Work out the finished part from the listing and answer in its coordinate system (mm). Face numbers are marked on the shaded views. A direction names the side the tool comes from. Coordinates: 2 decimals unless noted, no trailing zeros. Order: outer loops, then holes, each group sorted by start corner. A loop starts at its lowest first (then second) coordinate and runs counter-clockwise, first axis right, second up.
Autodesk Inventor part; units mm, degrees
ref_plane "YZ Plane" through (0, 0, 0) normal (1, 0, 0) x (0, 1, 0)
ref_plane "XZ Plane" through (0, 0, 0) normal (0, 1, 0) x (-1, 0, 0)
ref_plane "XY Plane" through (0, 0, 0) normal (0, 0, 1) x (1, 0, 0)
sketch "Sketch1" plane through (0, 0, 0) normal (0, 1, 0) x (-1, 0, 0)
  line L0 (0, 0) -> (1000, 0)
  line L1 (1000, 0) -> (1000, 1000)
  line L2 (1000, 1000) -> (0, 1000)
  line L3 (0, 1000) -> (0, 0)
  line L4 (-100, 1100) -> (1100, 1100)
  line L5 (1100, 1100) -> (1100, -100)
  line L6 (1100, -100) -> (-100, -100)
  line L7 (-100, -100) -> (-100, 1100)
  dimension "d0" = 1000
  dimension "d1" = 1000
  dimension "d2" = 100
extrude "Extrusion1" add sketch "Sketch1" along normal blind 850 contours L3 L2 L1 L0
extrude "Extrusion2" add sketch "Sketch1" along normal blind 10
sketch "Sketch2" plane through (0, 10, 0) normal (0, 1, 0) x (1, 0, 0)
  line L0 (100, 100) -> (-1100, 100)
  line L1 (-1100, 100) -> (-1100, -1100)
  line L2 (-1100, -1100) -> (100, -1100)
  line L3 (100, -1100) -> (100, 100)
  line L4 (0, -1000) -> (0, 0)
  line L5 (-1000, -1000) -> (0, -1000)
  line L6 (-1000, 0) -> (-1000, -1000)
  line L7 (0, 0) -> (-1000, 0)
  line L8 (-1000, -1000) -> (-1050, -1000)
  line L9 (-1050, -1000) -> (-1050, -1050)
  line L10 (-1050, -1050) -> (50, -1050)
  line L11 (50, -1050) -> (50, 50)
  line L12 (50, 50) -> (-1050, 50)
  line L13 (-1050, 50) -> (-500, 50)
  line L14 (-500, 50) -> (-500, -1050)
  line L15 (50, 50) -> (50, -500)
  line L16 (50, -500) -> (-1000, -500)
  line L17 (-1000, -500) -> (-1050, -500)
  dimension "d7" = 50
  dimension "d8" = 50
  dimension "d9" = 1100
  dimension "d10" = 1100
  dimension "d11" = 550
hole "Hole1" at (-1050, 10, 1050) at (-500, 10, 1050) at (50, 10, 1050) at (50, 10, -50) at (-500, 10, -50) at (-1050, 10, -50) at (50, 10, 500) at (-1050, 10, 500) direction (0, -1, 0) diameter 25.4 end through all
sketch "Sketch3" plane through (0, 850, 1000) normal (1, 0, 0) x (0, 0, -1)
  line L0 (0, -59.4954) -> (1000, -59.4954) construction
  line L1 (1000, -59.4954) -> (1000, -749.3909) construction
  line L2 (1000, -749.3909) -> (0, -749.3909) construction
  line L3 (0, -749.3909) -> (0, -59.4954) construction
  point P0 (1000, -850)
decal "Decal1"
sketch "Sketch4" plane through (-1000, 850, 1000) normal (0, 0, 1) x (1, 0, 0)
  line L0 (0, -840) -> (0, 0)
  line L1 (0, -64.0631) -> (1000, -64.0631) construction
  line L2 (1000, -64.0631) -> (1000, -753.9585) construction
  line L3 (1000, -753.9585) -> (0, -753.9585) construction
  line L4 (0, -753.9585) -> (0, -64.0631) construction
  point P0 (1000, -850)
decal "Decal2"
sketch "Sketch5" plane through (-1000, 850, 0) normal (-1, 0, 0) x (0, 0, 1)
  line L0 (57.8435, -18.5187) -> (921.1484, -18.5187) construction
  line L1 (921.1484, -18.5187) -> (921.1484, -825.537) construction
  line L2 (921.1484, -825.537) -> (57.8435, -825.537) construction
  line L3 (57.8435, -825.537) -> (57.8435, -18.5187) construction
  point P0 (0, -850)
decal "Decal3"
sketch "Sketch6" plane through (0, 850, 0) normal (0, 0, -1) x (-1, 0, 0)
  line L0 (-2.3743, -103.2912) -> (997.1946, -103.2912) construction
  line L1 (997.1946, -103.2912) -> (997.1946, -725.2451) construction
  line L2 (997.1946, -725.2451) -> (-2.3743, -725.2451) construction
  line L3 (-2.3743, -725.2451) -> (-2.3743, -103.2912) construction
  point P0 (0, -850)
decal "Decal4"
sketch "Sketch7" plane through (0, 0, 0) normal (0, -1, 0) x (1, 0, 0)
  circle A0 centre (-1050, 500) radius 12.7
  circle A1 centre (-500, 500) radius 5
  point P0 (0, 0)
  dimension "d73" = 10
extrude "Extrusion3" cut sketch "Sketch7" against normal blind 1 contours A1
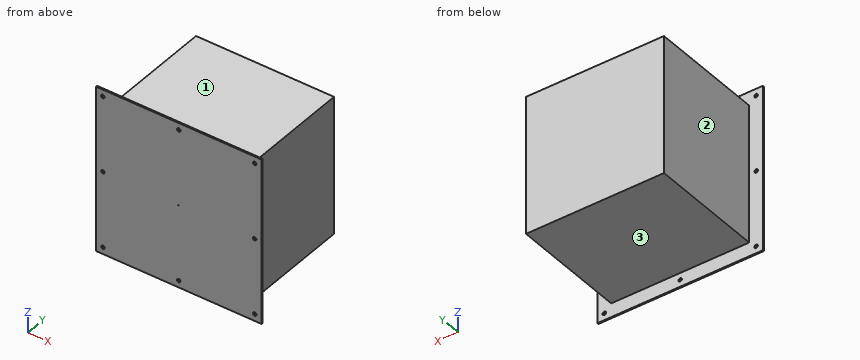
1. The part is cut by section B-B (x = -468.5). Determine the outline of the cut face in (y, z).
2. The part is cut by section A-A (z = 537). Determine the outline of the cut face in (x, y), plus the area to 3 significant figures.
3. The part is cut by section C-C (y = 680). Determine the outline of the cut face in (x, z).
4. Flat-ended cylindrical pins translate along their axes: pin 1 (5 mm diameter, centred on x = -500.5, z = 499.5, fed in from -Y); pin 2 (1 mm diameter, centred on y = 151.5, z = 502, fed in from +X); pin 3 (1 mm diameter, centred on y = 742.5, z = 599, fed in from -X); pin 4 (10 mm diameter, centred on x = -564.5, z = 737.5, fed in from -Y). Find the tip coordinate at first contact, or state that the pin passes through.
5. Consider probe 1 along Z at (x, y) = (-500, 8); probe 2 along Z at (x, y) = (-1050, 5); probe 3 along X at (y, z) = (3.5, -50). Determine where each line is inside the solid, lowest interval first.
6. For the marked faces 1, 2 and 3, determine the directions among +Z, -Z, +X, -X, +Y, -Y from which every point of the face is accessible in a straight line to the end or side of a thin tool.
Worked out:
1. outline: (0, -100) - (10, -100) - (10, 0) - (850, 0) - (850, 1000) - (10, 1000) - (10, 1100) - (0, 1100) - close
2. outline: (-1100, 0) - (100, 0) - (100, 10) - (0, 10) - (0, 850) - (-1000, 850) - (-1000, 10) - (-1100, 10) - close
2. area: 852,000 mm2
3. outline: (-1000, 0) - (0, 0) - (0, 1000) - (-1000, 1000) - close
4. pin 1: stops at y = 1
4. pin 2: stops at x = 0
4. pin 3: stops at x = -1000
4. pin 4: stops at y = 0
5. probe 1: z = -100 to -62.7, -37.3 to 1037.3, 1062.7 to 1100
5. probe 2: z = -100 to -62.7, -37.3 to 487.3, 512.7 to 1037.3, 1062.7 to 1100
5. probe 3: x = -1100 to -1062.7, -1037.3 to -512.7, -487.3 to 37.3, 62.7 to 100
6. face 1: +Z, +X, -X, +Y
6. face 2: +Z, -Z, -X, +Y
6. face 3: -Z, +X, -X, +Y
